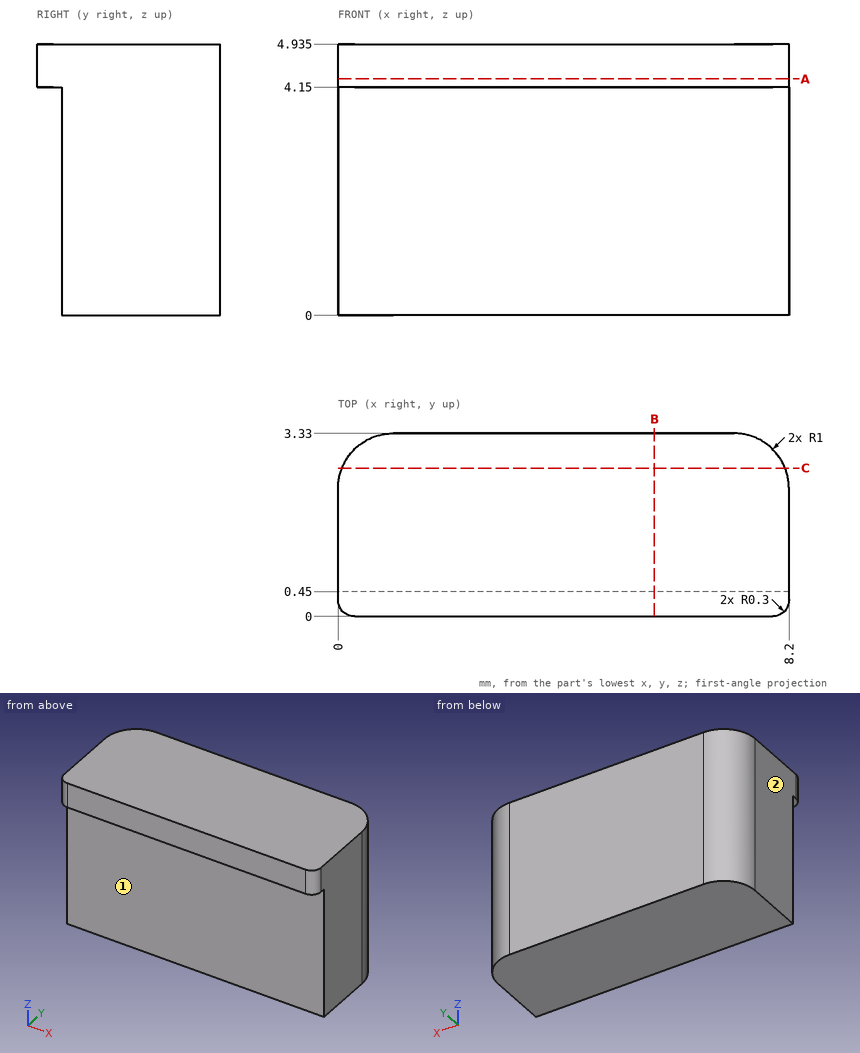
Answer from the drawing. Dimensions are ordinates in mm from the lowest x, y and z of the part. A direction names the side the tool comes from. Give positions to 0.01 mm unless a question says otherwise; leave off trailing zeros. Write each loop counter-clockwise with the first axis right and the second up, starting at its lowest first coordinate (ties: lowest second). Pieces come first, ordered by that corner, then holes. Notation, with made-up numbers: (14, 16.5) - (32, 16.5) arc R33 cw to (32, 46.5) - close; hole circle Ø3 at (83.25, 85.5). An arc over 180 degrees is marked (long way). One line per item, written item: value. Start each with the question number.
1. Find section B-B (x = 5.75). Write down the section's boundary in (y, z) (3 decimals), then the cut area to 3 significant figures.
2. Consider probe 1 along Y at (x, z) = (1.25, 1.1); probe 2 along Z at (x, y) = (4.25, 0.4) (3 decimals); probe 3 along X at (y, z) = (2.4, 0.4). Determine where each line is inside the solid, lowest interval first.
3. Find section C-C (y = 2.7). Write down the section's boundary in (x, z) (3 decimals), then the cut area to 3 significant figures.
4. For the marked faces 1 and 2, determine the directions among +Z, -Z, +X, -X, +Y, -Y from which every point of the face is accessible in a straight line to the end or side of a thin tool.
5. Find section A-A (z = 4.3). Write down the section's boundary in (x, y).
6. Given pin 1 (2 mm diameter, centred on x = 6, z = 2, fed in from -Y); pin 2 (1 mm diameter, centred on y = 2, z = 3, fed in from -X), each flat-ended and moving along its own axis, determine where each tip first touches the part or whether it passes through.
Geometry results:
1. outline: (0, 4.15) - (0.45, 4.15) - (0.45, 0) - (3.33, 0) - (3.33, 4.935) - (0, 4.935) - close
1. area: 14.6 mm2
2. probe 1: 0.45 to 3.33
2. probe 2: 4.15 to 4.935
2. probe 3: 0 to 8.2
3. outline: (0.071, 0) - (8.129, 0) - (8.129, 4.935) - (0.071, 4.935) - close
3. area: 39.8 mm2
4. face 1: -Z, +X, -X, -Y
4. face 2: +Z, -Z, -X, +Y, -Y
5. outline: (0, 0.3) arc R0.3 ccw to (0.3, 0) - (7.9, 0) arc R0.3 ccw to (8.2, 0.3) - (8.2, 2.33) arc R1 ccw to (7.2, 3.33) - (1, 3.33) arc R1 ccw to (0, 2.33) - close
6. pin 1: y = 0.45
6. pin 2: x = 0
